from build123d import *

# Parameters (mm, degrees)
CROQUIS1_W            = 17
CROQUIS1_H            = 4
EXTRUIR1_DEPTH        = 8.4
CORTAR_EXTRUIR1_DEPTH = 5.4
CHAFL_N1_SIZE         = 0.6
EXTRUIR2_DEPTH        = 5.4
CHAFL_N2_SIZE         = 0.3


with BuildPart() as part:
    # Croquis1 → Extruir1 (new body)
    with BuildSketch(Plane(origin=(0, 0, 0), x_dir=(1, 0, 0), z_dir=(0, 1, 0))):
        Rectangle(CROQUIS1_W, CROQUIS1_H)
    extrude(amount=EXTRUIR1_DEPTH)

    # Croquis2 → Cortar-Extruir1 (cut)
    with BuildSketch(Plane(origin=(0, 8.4, 0), x_dir=(-1, 0, 0), z_dir=(0, 1, 0))):
        Polygon((-6.8, -2), (6.5, -2), (6.5, -1.2), (7.5, -1.2), (7.5, 1.2), (6.5, 1.2), (6.5, 2), (-6.8, 2), align=None)
    extrude(amount=-CORTAR_EXTRUIR1_DEPTH, mode=Mode.SUBTRACT)

    # Chaflán1
    chafl_n1_edges = [part.edges().sort_by_distance(p)[0] for p in [
        (6.8, 8.4, 0),
        (-6.5, 8.4, -1.6),
        (-6.5, 8.4, 1.6),
    ]]
    chamfer(chafl_n1_edges, length=CHAFL_N1_SIZE)

    # Croquis3 → Extruir2 (add)
    with BuildSketch(Plane(origin=(0, 3, 0), x_dir=(-1, 0, 0), z_dir=(0, 1, 0))):
        Polygon((-5, -1.15), (-5, 1.15), (5, 1.15), (5, -0.15), (-3.7, -0.15), (-3.7, -1.15), align=None)
    extrude(amount=EXTRUIR2_DEPTH)

    # Chaflán2
    chafl_n2_edges = [part.edges().sort_by_distance(p)[0] for p in [
        (4.35, 8.4, -1.15),
        (3.7, 8.4, -0.65),
        (-0.65, 8.4, -0.15),
        (-5, 8.4, 0.5),
        (0, 8.4, 1.15),
        (5, 8.4, 0),
    ]]
    chamfer(chafl_n2_edges, length=CHAFL_N2_SIZE)


solid = part.part
Build history of the part. All positions in model axes, mm. A direction names the side the tool comes from. Round coordinates to 2 decimals unless told otherwise and drop trailing zeros. Loops run counter-clockwise (first coordinate to the right, second up) from the corner with the lowest first, then second, coordinate; pieces in that order, holes last. Notation, with made-up numbers: (-12.5, -27) -> (38.5, -27) arc R14 ccw to (38.5, 0) -> close; hole circle Ø1 at (-5, 47.5). An arc over 180 degrees is marked (long way). One line per item, written item: value. Start each with the question number.
Q1. Cut at A-A on y = 4. List the corners of the cut face in (x, z).
Q2. Cut at D-D on z = -0.65. List the corners of the cut face in (x, y), plus the area to 3 significant figures.
Q3. Cut at B-B on x = -0.75. List the corners of the cut face in (y, z).
Q4. Two-plate mould, pull along Z, no slides. Class faces 1 (the face through (-7, 6, 1.2)), 2 (the face through (-1, 6, -0.15)), 3 (the face through (0, 2, 2)): released by +Z, released by -Z, zero draft, split by the parting line, or undercut.
Q5. Probe line 1 along X through (y, z) = (6.75, 0.65); line 2 along X through (y, z) = (3.75, 1.3); line 3 along Y through (x, z) = (6.75, 0.45). List the from-to ranges inside material, lowest first.
Q6. Drop flat-ended pins along their axis: pin 1 Ø2 at (x, y) = (-5, 4.5) entering from -Z; pin 2 Ø0.6 at (x, y) = (4, 4.5) entering from -Z. Give the stop position or say it passes through.
Q7. 3-axis set-ups, long thin cutter, end or side, ignore diameter. For faces 4 (the face through (-7.5, 6, 0)), 5 (the face through (4, 6, -1.15)), 6 (the face through (6.8, 5, 0)): which of +Z, -Z, +X, -X, +Y, -Y reach the whole face in a straight line?
Q8. Cut at C-C on z = 0.45. List the corners of the cut face in (x, y), plus the area to 3 significant figures.
Computed:
1. outline: (-8.5, -2) -> (-6.5, -2) -> (-6.5, -1.2) -> (-7.5, -1.2) -> (-7.5, 1.2) -> (-6.5, 1.2) -> (-6.5, 2) -> (-8.5, 2) -> close; (-5, -0.15) -> (3.7, -0.15) -> (3.7, -1.15) -> (5, -1.15) -> (5, 1.15) -> (-5, 1.15) -> close; (6.8, -2) -> (8.5, -2) -> (8.5, 2) -> (6.8, 2) -> close
2. outline: (-8.5, 0) -> (8.5, 0) -> (8.5, 8.4) -> (7.4, 8.4) -> (6.8, 7.8) -> (6.8, 3) -> (5, 3) -> (5, 8.1) -> (4.7, 8.4) -> (4, 8.4) -> (3.7, 8.1) -> (3.7, 3) -> (-7.5, 3) -> (-7.5, 8.4) -> (-8.5, 8.4) -> close
2. area: 72.3 mm²
3. outline: (0, -2) -> (3, -2) -> (3, -0.15) -> (8.1, -0.15) -> (8.4, 0.15) -> (8.4, 0.85) -> (8.1, 1.15) -> (3, 1.15) -> (3, 2) -> (0, 2) -> close
4. face 1: undercut
4. face 2: released by -Z
4. face 3: released by +Z
5. line 1: -8.5 to -7.5, -5 to 5, 6.8 to 8.5
5. line 2: -8.5 to -6.5, 6.8 to 8.5
5. line 3: 0 to 3
6. pin 1: z = -0.15
6. pin 2: z = -1.15
7. face 4: +Y
7. face 5: -Z, +Y
7. face 6: +Z, -Z, +Y
8. outline: (-8.5, 0) -> (8.5, 0) -> (8.5, 8.4) -> (7.4, 8.4) -> (6.8, 7.8) -> (6.8, 3) -> (5, 3) -> (5, 8.1) -> (4.7, 8.4) -> (-4.7, 8.4) -> (-5, 8.1) -> (-5, 3) -> (-7.5, 3) -> (-7.5, 8.4) -> (-8.5, 8.4) -> close
8. area: 119 mm²
